Can you work these out from the drawing? Everything is in mm from the part's minimum corner. Round coordinates to 2 decimals unless told otherwise and drop trailing zeros. Write each loop counter-clockwise with the first axis right and the second up, starting at its lowest first coordinate (ties: lowest second). Pieces come first, ordered by that corner, then holes.
Q1. Please list where these lines run through material, in increasing order: line 1 along Y through (x, z) = (18, 2.5); line 2 along X through (y, z) = (19, 3.3); line 3 along X through (y, z) = (8, 1.6).
Q2. If we section it at C-C (z = 4.45): Please give me the cut outline in (x, y), plus the area to 4 significant figures.
Q3. If we section it at D-D (x = 11.5): Please give me the cut outline in (y, z).
Q4. I'm going to push flat-ended pins straight in: pin 1 Ø2 at (y, z) = (14, 1) entering from -X; pin 2 Ø1.5 at (x, z) = (32, 4) entering from +Y; pin 3 Ø1.5 at (x, z) = (24, 2.5) entering from -Y. Where does each tip first touch, or does it pass through?
Q5. If we section it at A-A (y = 18): Please give me the cut outline in (x, z), plus the area to 4 significant figures.
Q6. We'd pull the mould along Y, two halves only. Please class the marked faces 1, 2 and 3: +Y half, -Y half, draft (parallel to the pull), parting line (faces both ways), or undercut.
Q7. If we section it at B-B (x = 18): Please give me the cut outline in (y, z), plus the area to 4 significant figures.
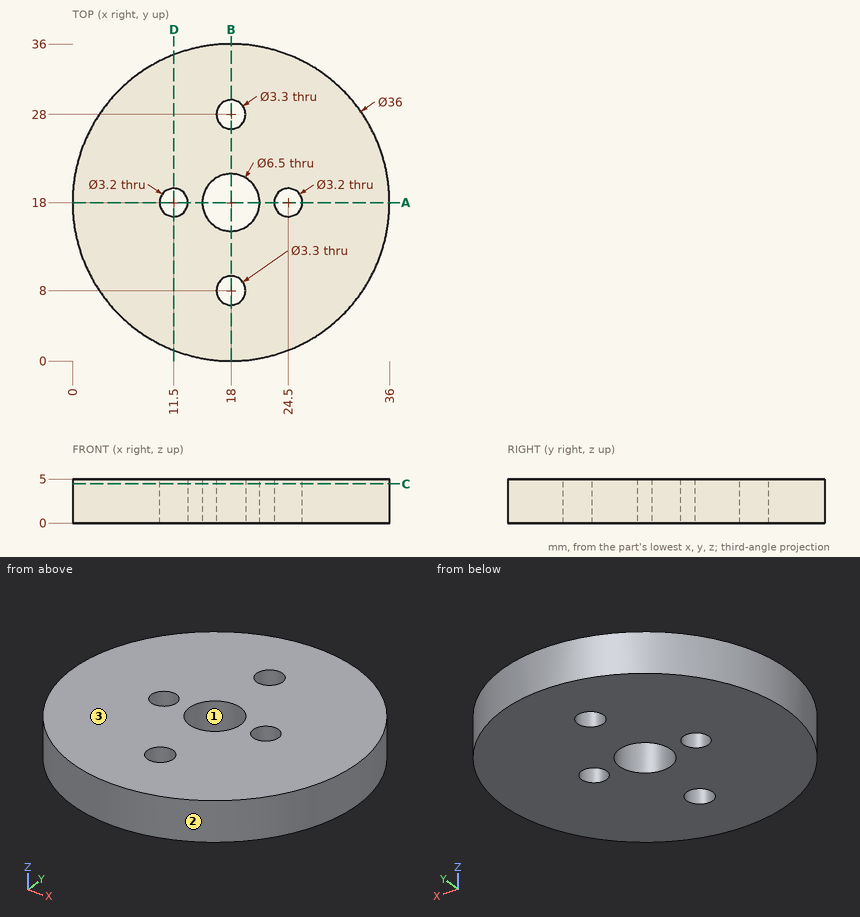
A:
1. line 1: y = 0 to 6.35, 9.65 to 14.75, 21.25 to 26.35, 29.65 to 36
1. line 2: x = 0.03 to 10.25, 12.75 to 14.91, 21.09 to 23.25, 25.75 to 35.97
1. line 3: x = 3.03 to 16.35, 19.65 to 32.97
2. outline: circle Ø36 at (18, 18); hole circle Ø3.2 at (11.5, 18); hole circle Ø6.5 at (18, 18); hole circle Ø3.3 at (18, 8); hole circle Ø3.3 at (18, 28); hole circle Ø3.2 at (24.5, 18)
2. area: 951.5 mm2
3. outline: (1.21, 0) - (16.4, 0) - (16.4, 5) - (1.21, 5) - close; (19.6, 0) - (34.79, 0) - (34.79, 5) - (19.6, 5) - close
4. pin 1: stops at x = 0.25
4. pin 2: stops at y = 30.18
4. pin 3: stops at y = 0.78
5. outline: (0, 0) - (9.9, 0) - (9.9, 5) - (0, 5) - close; (13.1, 0) - (14.75, 0) - (14.75, 5) - (13.1, 5) - close; (21.25, 0) - (22.9, 0) - (22.9, 5) - (21.25, 5) - close; (26.1, 0) - (36, 0) - (36, 5) - (26.1, 5) - close
5. area: 115.5 mm2
6. face 1: undercut
6. face 2: parting line
6. face 3: draft
7. outline: (0, 0) - (6.35, 0) - (6.35, 5) - (0, 5) - close; (9.65, 0) - (14.75, 0) - (14.75, 5) - (9.65, 5) - close; (21.25, 0) - (26.35, 0) - (26.35, 5) - (21.25, 5) - close; (29.65, 0) - (36, 0) - (36, 5) - (29.65, 5) - close
7. area: 114.5 mm2
